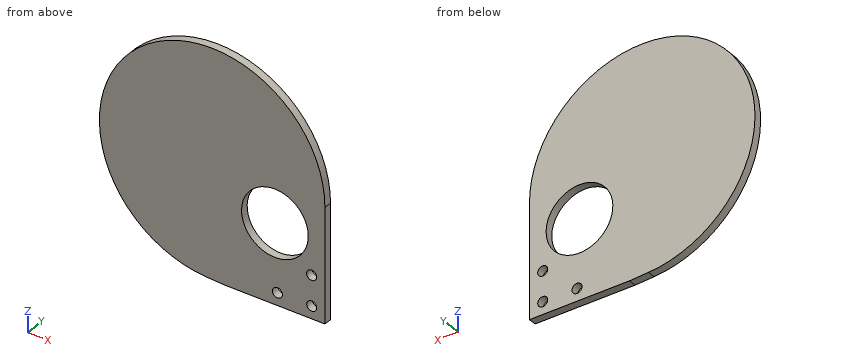
from build123d import *

# Parameters (mm, degrees)
SKETCH1_R           = 13.335
BOSS_EXTRUDE1_DEPTH = 3.175
CUT_EXTRUDE1_REACH  = 93.585
SKETCH2_R           = 2


with BuildPart() as part:
    # Sketch1 → Boss-Extrude1 (new body)
    with BuildSketch(Plane(origin=(0, 0, 0), x_dir=(1, 0, 0), z_dir=(0, 1, 0))):
        with BuildLine():
            Line((-20.000000005, 31.75), (-27.57263297, 31.331531049))
            ThreePointArc((-27.57263297, 31.331531049), (-56.072919353, -46.432398987), (20.000000005, -13.684787183))
            Line((20.000000005, -13.684787183), (20.000000005, 31.75))
            Line((20.000000005, 31.75), (-20.000000005, 31.75))
        make_face()
        with Locations(Location((0, 0, 0), (0, 0, 270))):
            Circle(SKETCH1_R, mode=Mode.SUBTRACT)
    extrude(amount=BOSS_EXTRUDE1_DEPTH)

    # Sketch2 → Cut-Extrude1 (cut, up to next)
    with BuildSketch(Plane.XZ, mode=Mode.PRIVATE) as cut_extrude1_sk1:
        with Locations(Location((14.706006433, -14.75, 0), (0, 0, 270))):
            Circle(SKETCH2_R)
    cut_extrude1_tool1 = extrude(cut_extrude1_sk1.sketch, amount=-CUT_EXTRUDE1_REACH, mode=Mode.PRIVATE) & part.part
    # Sketch2 → Cut-Extrude1 (cut, up to next)
    with BuildSketch(Plane.XZ, mode=Mode.PRIVATE) as cut_extrude1_sk2:
        with Locations(Location((14.706006433, -26.75, 0), (0, 0, 270))):
            Circle(SKETCH2_R)
    cut_extrude1_tool2 = extrude(cut_extrude1_sk2.sketch, amount=-CUT_EXTRUDE1_REACH, mode=Mode.PRIVATE) & part.part
    # Sketch2 → Cut-Extrude1 (cut, up to next)
    with BuildSketch(Plane.XZ, mode=Mode.PRIVATE) as cut_extrude1_sk3:
        with Locations(Location((1, -26.75, 0), (0, 0, 270))):
            Circle(SKETCH2_R)
    cut_extrude1_tool3 = extrude(cut_extrude1_sk3.sketch, amount=-CUT_EXTRUDE1_REACH, mode=Mode.PRIVATE) & part.part
    add(cut_extrude1_tool1.solids().sort_by_distance((14.706006, 0, -14.75))[0], mode=Mode.SUBTRACT)
    add(cut_extrude1_tool2.solids().sort_by_distance((14.706006, 0, -26.75))[0], mode=Mode.SUBTRACT)
    add(cut_extrude1_tool3.solids().sort_by_distance((1, 0, -26.75))[0], mode=Mode.SUBTRACT)


solid = part.part
Design review of the part built by this model. Coordinates are the model's own, in mm. Round coordinates to 2 decimals unless told otherwise and drop trailing zeros. Loops run counter-clockwise (first coordinate to the right, second up) from the corner with the lowest first, then second, coordinate; pieces in that order, holes last. Notation, with made-up numbers: (-31, -37.5) - (-7, -37.5) arc R18 cw to (-7, -31.5) - close; hole circle Ø8 at (89.5, -6). An arc over 180 degrees is marked (long way). One line per item, written item: value. Start each with the question number.
1) Consider section D-D on y = 0.9. Give the boundary of the cut face in (x, z) (3 decimals).
2) To check wall thickness, follow L1, parallel to X at y = 2.55, z = -26.75; L2, parallel to X at y = 2.1, z = 7.5; L3, parallel to X at y = 1.2, z = 9. State the ranges of each line that lie inside material, in increasing order. Write a range as from..to.
3) Consider section A-A on x = 5. Give the boundary of the cut face in (y, z) (3 decimals), then the cut area to 3 significant figures.
4) Insertion check: pin 1 Ø6.5 at (x, z) = (14.71, -26.75) entering from -Y; pin 2 Ø1 at (y, z) = (2.5, -11) entering from -X. Each pin has a flat end and moves straight along its axis. Give the tip position at first contact, or say it passes through.
5) Consider section C-C on z = 0. Give the boundary of the cut face in (x, y) (3 decimals), then the cut area to 3 significant figures.
6) Consider section B-B on z = -26.75. Give the boundary of the cut face in (x, y) (3 decimals).
Reported:
1. outline: (-27.573, -31.332) - (-20, -31.75) - (20, -31.75) - (20, 13.685) arc R45.085 ccw (long way) to start; hole circle Ø26.67 at (0, 0); hole circle Ø4 at (1, -26.75); hole circle Ø4 at (14.706, -26.75); hole circle Ø4 at (14.706, -14.75)
2. L1: x = -45.03..-1, 3..12.71, 16.71..20
2. L2: x = -69.74..-11.03, 11.03..20
2. L3: x = -69.93..-9.84, 9.84..20
3. outline: (0, -31.75) - (3.175, -31.75) - (3.175, -12.362) - (0, -12.362) - close; (0, 12.362) - (3.175, 12.362) - (3.175, 47.264) - (0, 47.264) - close
3. area: 172 mm^2
4. pin 1: stops at y = 0
4. pin 2: stops at x = -63.13
5. outline: (-68.043, 0) - (-13.335, 0) - (-13.335, 3.175) - (-68.043, 3.175) - close; (13.335, 0) - (20, 0) - (20, 3.175) - (13.335, 3.175) - close
5. area: 195 mm^2
6. outline: (-45.027, 0) - (-1, 0) - (-1, 3.175) - (-45.027, 3.175) - close; (3, 0) - (12.706, 0) - (12.706, 3.175) - (3, 3.175) - close; (16.706, 0) - (20, 0) - (20, 3.175) - (16.706, 3.175) - close
